```python
from build123d import *

# Parameters (mm, degrees)
SKETCH_1_R          = 22.5
EXTRUDE_1_DEPTH     = 12
SKETCH_2_R          = 4.2
CUT_EXTRUDE_1_DEPTH = 4.4
SKETCH_3_R          = 2.6
CUT_EXTRUDE_2_DEPTH = 35.007352146
SKETCH_4_R          = 4
CUT_EXTRUDE_3_DEPTH = 35.007352146
SKETCH_5_R          = 11
CUT_EXTRUDE_4_DEPTH = 35.007352146


with BuildPart() as part:
    # 草图1 → 凸台-拉伸1 (new body)
    with BuildSketch(Plane(origin=(0, 0, 0), x_dir=(1, 0, 0), z_dir=(0, 1, 0))):
        with Locations(Location((0, 0, 0), (0, 0, 270))):
            Circle(SKETCH_1_R)
    extrude(amount=EXTRUDE_1_DEPTH)

    # 草图2 → 切除-拉伸1 (cut)
    with BuildSketch(Plane.XZ):
        with Locations(Location((17.5, 0, 0), (0, 0, 270))):
            Circle(SKETCH_2_R)
        with Locations(Location((0, 17.5, 0), (0, 0, 270))):
            Circle(SKETCH_2_R)
        with Locations(Location((-17.5, 0, 0), (0, 0, 270))):
            Circle(SKETCH_2_R)
        with Locations(Location((0, -17.5, 0), (0, 0, 270))):
            Circle(SKETCH_2_R)
    extrude(amount=-CUT_EXTRUDE_1_DEPTH, mode=Mode.SUBTRACT)

    # 草图3 → 切除-拉伸2 (cut, through all)
    with BuildSketch(Plane.XZ):
        with Locations(Location((0, 17.5, 0), (0, 0, 270))):
            Circle(SKETCH_3_R)
        with Locations(Location((17.5, 0, 0), (0, 0, 270))):
            Circle(SKETCH_3_R)
        with Locations(Location((0, -17.5, 0), (0, 0, 270))):
            Circle(SKETCH_3_R)
        with Locations(Location((-17.5, 0, 0), (0, 0, 270))):
            Circle(SKETCH_3_R)
    extrude(amount=-CUT_EXTRUDE_2_DEPTH, mode=Mode.SUBTRACT)

    # 草图4 → 切除-拉伸3 (cut, through all)
    with BuildSketch(Plane.XZ):
        with Locations(Location((0, 0, 0), (0, 0, 270))):
            Circle(SKETCH_4_R)
    extrude(amount=-CUT_EXTRUDE_3_DEPTH, mode=Mode.SUBTRACT)

    # 草图5 → 切除-拉伸4 (cut, through all)
    with BuildSketch(Plane.XZ):
        with Locations(Location((0, 0, 0), (0, 0, 270))):
            Circle(SKETCH_5_R)
    extrude(amount=-CUT_EXTRUDE_4_DEPTH, mode=Mode.SUBTRACT)


solid = part.part
```
The model under review builds one solid part; all positions refer to its coordinate system, in mm. A direction names the side the tool comes from. Round coordinates to 2 decimals unless told otherwise and drop trailing zeros. Write each loop counter-clockwise with the first axis right and the second up, starting at its lowest first coordinate (ties: lowest second). Pieces come first, ordered by that corner, then holes. Notation, with made-up numbers: (50.5, 42.5) - (59.5, 42.5) arc R16 cw to (59.5, 67.5) - close; hole circle Ø1 at (-32.5, 39). An arc over 180 degrees is marked (long way). One line per question, with ' | ' between items.
Item 1: Add section B-B, the plane z = 5.5. Give the boundary of the cut face in (x, y).
Resolved:
outline: (-21.82, 0) - (-9.53, 0) - (-9.53, 12) - (-21.82, 12) - close; (9.53, 0) - (21.82, 0) - (21.82, 12) - (9.53, 12) - close
Item 2: The part is to be moulded in two halves that separate along Z. For faces 1 (the face through (5, 12, 10)), 2 (the face through (-8.618, 5.916, 20.784)), 3 (the face through (-10.74, 5.92, 2.38)), say which applies: pulls with the +Z half, pulls with the -Z half, needs draft (parallel to the pull), parting line crosses it, or undercut.
Resolved:
face 1: needs draft | face 2: parting line crosses it | face 3: undercut
Item 3: To check wall thickness, follow probe 1 along X at (y, z) = (2.2, 0); probe 2 along X at (y, z) = (7.25, 0); probe 3 along Z at (x, y) = (5, 9.25). State the ranges of each line that lie inside material, in increasing order.
Resolved:
probe 1: x = -22.5 to -21.7, -13.3 to -11, 11 to 13.3, 21.7 to 22.5 | probe 2: x = -22.5 to -20.1, -14.9 to -11, 11 to 14.9, 20.1 to 22.5 | probe 3: z = -21.94 to -9.8, 9.8 to 21.94
Item 4: Add section C-C, the plane y = 3.5. Give the boundary of the cut face in (x, z).
Resolved:
outline: circle Ø45 at (0, 0); hole circle Ø8.4 at (-17.5, 0); hole circle Ø22 at (0, 0); hole circle Ø8.4 at (0, -17.5); hole circle Ø8.4 at (0, 17.5); hole circle Ø8.4 at (17.5, 0)
Item 5: For P1, Ø4.5, axis at x = 17.5, z = 0, coming from the -Y side; P2, Ø2, axis at y = 4.5, z = -2, coming from the -X side; P3, Ø2, axis at x = 16, y = 3, coming from the -Z side; P4, Ø4, axis at x = -14.5, y = 7.5, coming from the -Z side, all flat-tipped, find the tip position at first contact; note any pin that passes through.
Resolved:
P1: passes through | P2: stops at x = -22.48 | P3: stops at z = -16.77 | P4: stops at z = -18.71
Item 6: Add section D-D, the plane z = 0. Give the boundary of the cut face in (x, y).
Resolved:
outline: (-22.5, 0) - (-21.7, 0) - (-21.7, 4.4) - (-20.1, 4.4) - (-20.1, 12) - (-22.5, 12) - close; (-14.9, 4.4) - (-13.3, 4.4) - (-13.3, 0) - (-11, 0) - (-11, 12) - (-14.9, 12) - close; (11, 0) - (13.3, 0) - (13.3, 4.4) - (14.9, 4.4) - (14.9, 12) - (11, 12) - close; (20.1, 4.4) - (21.7, 4.4) - (21.7, 0) - (22.5, 0) - (22.5, 12) - (20.1, 12) - close
Item 7: Add section A-A, the plane x = 0. Give the boundary of the cut face in (y, z).
Resolved:
outline: (0, -22.5) - (12, -22.5) - (12, -20.1) - (4.4, -20.1) - (4.4, -21.7) - (0, -21.7) - close; (0, -13.3) - (4.4, -13.3) - (4.4, -14.9) - (12, -14.9) - (12, -11) - (0, -11) - close; (0, 11) - (12, 11) - (12, 14.9) - (4.4, 14.9) - (4.4, 13.3) - (0, 13.3) - close; (0, 21.7) - (4.4, 21.7) - (4.4, 20.1) - (12, 20.1) - (12, 22.5) - (0, 22.5) - close
Item 8: For faces 4 (the face through (0.185, 2.169, 21.696)), 5 (the face through (0.78, 8.15, -19.98)), list the 3-axis set-ups (+Z, -Z, +X, -X, +Y, -Y) from which the entire face can be reached by the end or side of a thin tool; tool diameter is ignored.
Resolved:
face 4: -Y | face 5: +Y, -Y
